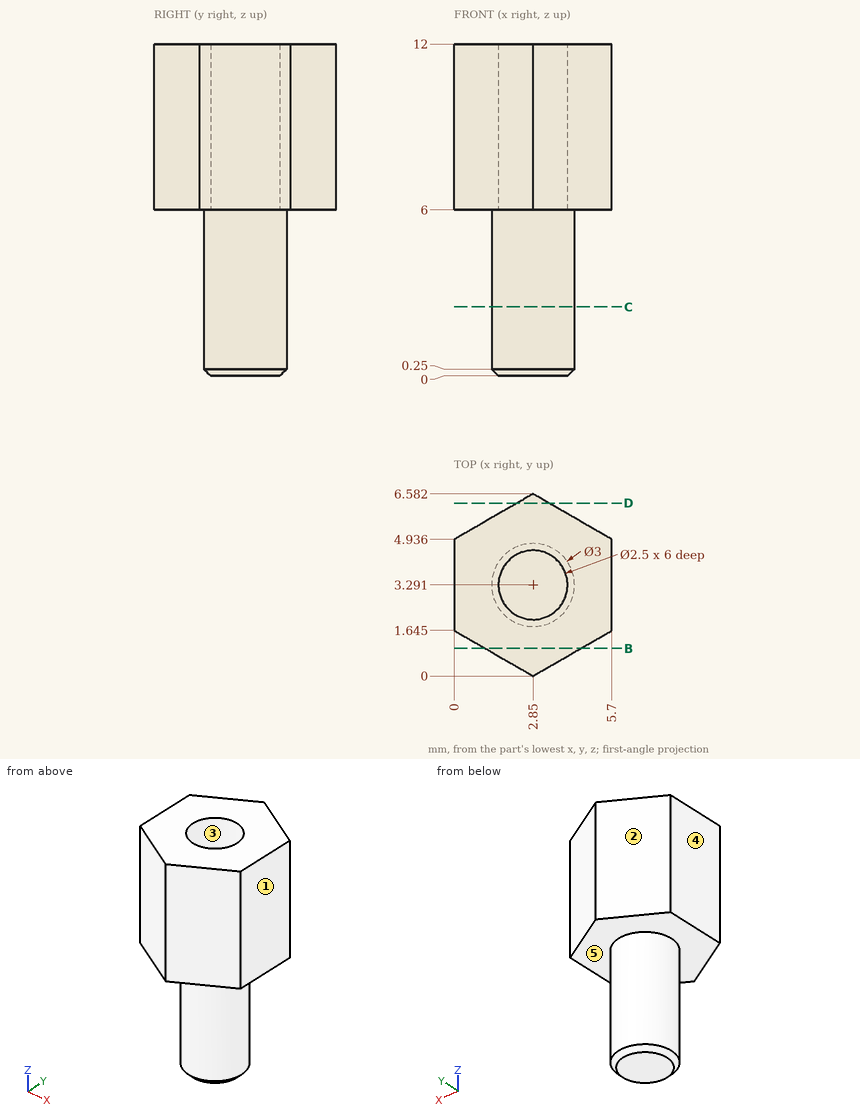
The drawing under review shows one solid part. Ordinate dimensions are in mm from its lowest x, y, z. A direction names the side the tool comes from. Round coordinates to 2 decimals unless told otherwise and drop trailing zeros. Loops run counter-clockwise (first coordinate to the right, second up) from the corner with the lowest first, then second, coordinate; pieces in that order, holes last.
Item 1: Mouldability with a two-part tool opening along X and no side actions: class the marked faces 1, 2 and 3 as released by +X, released by -X, zero draft, split by the parting line, or undercut.
Determined:
face 1: released by +X
face 2: released by -X
face 3: undercut
Item 2: Take a section at B-B (y = 1). Write out the cut boundary in (x, z), then the cut area to 3 significant figures.
Determined:
outline: (1.12, 6) - (4.58, 6) - (4.58, 12) - (1.12, 12) - close
area: 20.8 mm2
Item 3: Clearance check with a flat-ended pin moving along its axis: pin 1 Ø1.5 at (x, y) = (1, 5.5) entering from -Z. State where the tip first meets the part, or that it passes through.
Determined:
pin 1: stops at z = 6
Item 4: Take a section at D-D (y = 6.25). Write out the cut boundary in (x, z) (1 decimal).
Determined:
outline: (2.3, 6) - (3.4, 6) - (3.4, 12) - (2.3, 12) - close
Item 5: Take a section at C-C (z = 2.5). Write out the cut boundary in (x, y).
Determined:
outline: circle Ø3 at (2.85, 3.29)
Item 6: For the marked faces 4 and 5, list the 3-axis set-ups (+Z, -Z, +X, -X, +Y, -Y) from which the entire face can be reached by the end or side of a thin tool; tool diameter is ignored.
Determined:
face 4: +Z, -Z, -X, +Y, -Y
face 5: -Z
Item 7: For line 1 (X direction, y = 3.25, z = 10); line 2 (X direction, y = 4, z = 7); line 3 (Z direction, x = 0.6, y = 3.25), list the stretches that pass through material, from the lowest coordinate up.
Determined:
line 1: x = 0 to 1.6, 4.1 to 5.7
line 2: x = 0 to 1.82, 3.88 to 5.7
line 3: z = 6 to 12
